Check sheet for the modelled part. Datum: model origin and axes. Units: mm. Coordinates: 2 decimals unless noted, no trailing zeros. Order: outer loops, then holes, each group sorted by start corner. A loop starts at its lowest first (then second) coordinate and runs counter-clockwise, first axis right, second up.
1. Cross-section at B-B (z = -17.75). Enter the section's corners in (x, y), then the cut area to 3 significant figures.
2. Cross-section at C-C (y = 0.75). Enter the section's corners in (x, z).
3. Gauge pin test, flat ends, axial feed: pin 1 Ø2 at (x, z) = (-12, 3.5) entering from -Y; pin 2 Ø1.2 at (x, y) = (1, 0.5) entering from +Z; pin 3 Ø2 at (y, z) = (3.5, -12) entering from +X; pin 4 Ø1.6 at (x, y) = (1, 1) entering from -Z. Record the tip position at first contact, or that the pin passes through.
4. Thickness scan on line 1 (Z direction, x = -33.5, y = 1.1); line 2 (X direction, y = 1, z = 0); line 3 (Z direction, x = -57.25, y = 2.9). Record the ranges inside material, lowest first.
5. Cross-section at D-D (x = -33.5). Enter the section's corners in (y, z).
6. Cross-section at A-A (x = -63.75). Enter the section's corners in (y, z).
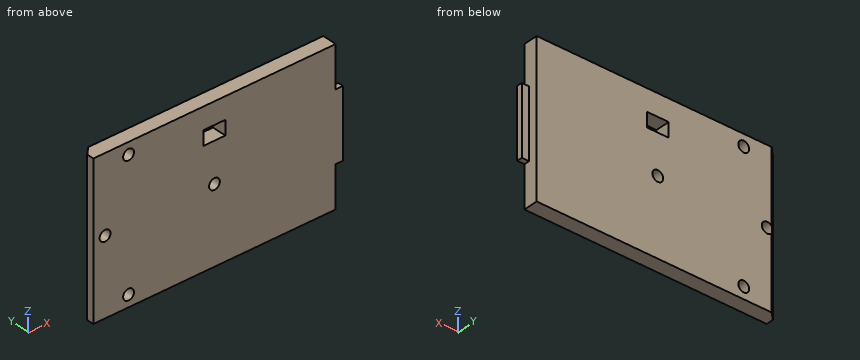
Autodesk Inventor part; units mm, degrees
ref_plane "YZ Plane" through (0, 0, 0) normal (1, 0, 0) x (0, 1, 0)
ref_plane "XZ Plane" through (0, 0, 0) normal (0, 1, 0) x (-1, 0, 0)
ref_plane "XY Plane" through (0, 0, 0) normal (0, 0, 1) x (1, 0, 0)
sketch "Sketch1" plane through (0, 0, 0) normal (0, 1, 0) x (-1, 0, 0)
  arc A0 (67, -23) -> (69, -21) centre (67, -21) ccw
  line L0 (69, -21) -> (69, 21)
  arc A1 (69, 21) -> (67, 23) centre (67, 21) ccw
  line L1 (67, 23) -> (0, 23)
  arc A2 (0, 23) -> (-2, 21) centre (0, 21) ccw
  line L2 (-2, 21) -> (-2, -21)
  arc A3 (-2, -21) -> (0, -23) centre (0, -21) ccw
  line L3 (0, -23) -> (67, -23)
  line L4 (67, -21) -> (0, -21)
  line L5 (0, -21) -> (0, 21)
  line L6 (0, 21) -> (67, 21)
  line L7 (67, 21) -> (67, -21)
  line L8 (67, 21) -> (60.5, 21)
  line L9 (60.5, 21) -> (60.5, 14.5)
  line L10 (60.5, 14.5) -> (67, 14.5)
  line L11 (67, 14.5) -> (67, 21)
  line L12 (67, -21) -> (67, 21)
  line L13 (67, -21) -> (60.5, -21)
  line L14 (60.5, -21) -> (60.5, -14.5)
  line L15 (60.5, -14.5) -> (67, -14.5)
  line L16 (67, -14.5) -> (67, -21)
  line L17 (67, -21) -> (60.5, -14.5)
  line L18 (67, 21) -> (69, 21)
  line L19 (67, 21) -> (60.5, 14.5)
  line L20 (0, 16.25) -> (-2, 16.25)
  circle A4 centre (64.5, -18.5) radius 1
  circle A5 centre (64.5, 18.5) radius 1
  line L21 (60.5, -21) -> (0, -21)
  line L22 (0, -21) -> (0, 21)
  line L23 (0, 21) -> (60.5, 21)
  line L24 (60.5, 21) -> (60.5, 14.5)
  line L25 (60.5, 14.5) -> (67, 14.5)
  line L26 (67, 14.5) -> (67, -14.5)
  line L27 (67, -14.5) -> (60.5, -14.5)
  line L28 (60.5, -14.5) -> (60.5, -21)
  arc A6 (67, -23) -> (69, -21) centre (67, -21) ccw
  line L29 (69, -21) -> (69, 21)
  arc A7 (69, 21) -> (67, 23) centre (67, 21) ccw
  line L30 (67, 23) -> (0, 23)
  arc A8 (0, 23) -> (-2, 21) centre (0, 21) ccw
  line L31 (-2, 21) -> (-2, -21)
  arc A9 (-2, -21) -> (0, -23) centre (0, -21) ccw
  line L32 (0, -23) -> (67, -23)
  line L33 (-2, -10) -> (0, -10)
  line L34 (0, -10) -> (0, 10)
  line L35 (0, 10) -> (-2, 10)
  line L36 (-2, 10) -> (-2, -10)
  line L37 (0, -21) -> (4.5, -21)
  line L38 (67, 21) -> (0, 21)
  line L39 (0, 21) -> (0, -21)
  line L40 (0, -21) -> (67, -21)
  line L41 (67, -21) -> (67, 21)
  line L42 (0, 16.25) -> (-2, 16.25)
  line L43 (67, -21) -> (60.5, -21)
  line L44 (0, -21) -> (0, 21)
  line L45 (0, 21) -> (54, 21)
  line L46 (67, 21) -> (67, 3.25)
  arc A10 (67, -23) -> (69, -21) centre (67, -21) ccw
  line L47 (69, -21) -> (69, 21)
  arc A11 (69, 21) -> (67, 23) centre (67, 21) ccw
  line L48 (67, 23) -> (0, 23)
  arc A12 (0, 23) -> (-2, 21) centre (0, 21) ccw
  line L49 (-2, 21) -> (-2, -21)
  arc A13 (-2, -21) -> (0, -23) centre (0, -21) ccw
  line L50 (0, -23) -> (67, -23)
  line L51 (-2, -10) -> (0, -10)
  line L52 (0, -10) -> (0, 10)
  line L53 (0, 10) -> (-2, 10)
  line L54 (-2, 10) -> (-2, -10)
  line L55 (0, -21) -> (4.5, -21)
  line L56 (67, 21) -> (0, 21)
  line L57 (0, 21) -> (0, -21)
  line L58 (0, -21) -> (67, -21)
  line L59 (67, -21) -> (67, 21)
  line L60 (60.5, -21) -> (60.5, -14.5)
  line L61 (60.5, -14.5) -> (54, -14.5)
  line L62 (54, -14.5) -> (54, -21)
  line L63 (54, -21) -> (0, -21)
  line L64 (54, 21) -> (54, 14.5)
  line L65 (54, 14.5) -> (60.5, 14.5)
  line L66 (60.5, 14.5) -> (60.5, 21)
  line L67 (60.5, 21) -> (67, 21)
  line L68 (67, 3.25) -> (60.5, 3.25)
  line L69 (60.5, 3.25) -> (60.5, -3.25)
  line L70 (60.5, -3.25) -> (67, -3.25)
  line L71 (67, -3.25) -> (67, -21)
  line L72 (67, -3.25) -> (60.5, 3.25)
  line L73 (54, -14.5) -> (60.5, -21)
  line L74 (54, 14.5) -> (60.5, 21)
  point P0 (0, 0)
  point P1 (0, 0)
  point P2 (0, 0)
  point P3 (0, 0)
  point P4 (63.75, 0)
  point P5 (57.25, -17.75)
  point P6 (57.25, 17.75)
  dimension "d0" = 6.5
  dimension "d1" = 6.5
  dimension "d2" = 6.5
  dimension "d3" = 6.5
  dimension "d4" = 10
  dimension "d5" = 10
  dimension "d25" = 10
  dimension "d26" = 10
extrude "Extrusion1" add sketch "Sketch1" along normal blind 2 contours L19 A5 L9 L6 | L7 L10 L19 A5 | L2 L35 L5 L33 | L74 L64 L6 | L9 L65 L74 | L7 L68 L69 L70 L15 L61 L62 L4 L5 L6 L64 L65 L10 | A5 L19 | L19 A5 | L7 L72 L68 | L70 L69 L72 | L7 L17 A4 L15 | L62 L73 L4 | L4 L14 L17 A4 | L14 L73 L61 | A4 L17 | L17 A4
sketch "Sketch2" plane through (0, 2, 0) normal (0, 1, 0) x (1, 0, 0)
  line L0 (0, -10) -> (2, -10)
  line L1 (2, -10) -> (2, 10)
  line L2 (2, 10) -> (0, 10)
  line L3 (0, 10) -> (0, 21)
  line L4 (0, 21) -> (-67, 21)
  line L5 (-67, 21) -> (-67, -21)
  line L6 (-67, -21) -> (0, -21)
  line L7 (0, -21) -> (0, -10)
  line L8 (-67, -21) -> (0, -21)
  line L9 (0, -21) -> (0, 21)
  line L10 (0, 21) -> (-67, 21)
  line L11 (-67, 21) -> (-67, -21)
  point P0 (0, 0)
extrude "Extrusion2" add sketch "Sketch2" along normal blind 2 contours L7 L6 L5 L4 L3 L9
sketch "Sketch3" plane through (-67, 0, 21) normal (0, 0, 1) x (1, 0, 0)
  point P0 (67, 0)
sketch "Sketch4" plane through (0, 4, 0) normal (0, 1, 0) x (1, 0, 0)
  line L0 (0, 21) -> (-67, 21)
  line L1 (-67, 21) -> (-67, -21)
  line L2 (-67, -21) -> (0, -21)
  line L3 (0, -21) -> (0, 21)
  line L4 (0, 10) -> (0, 21)
  line L5 (0, 21) -> (-67, -21)
  point P0 (0, 0)
  point P1 (-33.5, 0)
  point P2 (-57.25, 17.75)
  point P3 (-63.75, 0)
  point P4 (-57.25, -17.75)
  point P5 (-57.25, 17.75)
  point P6 (-63.75, 0)
  point P7 (-57.25, -17.75)
hole "Hole1" at (-33.5, 4, 0) at (-57.25, 4, -17.75) at (-57.25, 4, 17.75) at (-63.75, 4, 0) direction (0, -1, 0) diameter 3 depth 8 tip angle 118
sketch "Sketch5" plane through (2, 0, 10) normal (1, 0, 0) x (0, 0, -1)
  line L0 (0, 0) -> (20, 0)
  line L1 (20, 0) -> (20, 2)
  line L2 (0, 2) -> (20, 2)
  line L3 (0, 0) -> (0, 2)
  line L4 (20, 2) -> (20, 0)
  line L5 (20, 0) -> (0, 0)
  line L6 (0, 0) -> (0, 2)
  line L7 (0, 2) -> (20, 2)
  line L8 (0, 0) -> (20, 0)
  line L9 (0.5, 0) -> (19.5, 0)
  line L10 (19.5, 0) -> (19.5, 1.5)
  line L11 (19.5, 1.5) -> (0.5, 1.5)
  line L12 (0.5, 1.5) -> (0.5, 0)
  point P0 (10, 0)
  dimension "d20" = 0.5
  dimension "d21" = 0.5
  dimension "d22" = 0.5
extrude "Extrusion4" cut sketch "Sketch5" against normal up to surface (2 mm away) contours L3 L2 L1 L0 L10 L11 L12
sketch "Sketch6" plane through (0, 0, 0) normal (0, -1, 0) x (1, 0, 0)
  line L0 (-30.5, 15) -> (-36.5, 15)
  line L1 (-36.5, 15) -> (-36.5, 11)
  line L2 (-36.5, 11) -> (-30.5, 11)
  line L3 (-30.5, 11) -> (-30.5, 15)
  circle A0 centre (-63.75, 0) radius 1.5
  circle A1 centre (-57.25, -17.75) radius 1.5
  circle A2 centre (-33.5, 0) radius 1.5
  circle A3 centre (-57.25, 17.75) radius 1.5
  line L4 (2, 9.5) -> (0, 9.5)
  line L5 (0, 21) -> (0, 9.5)
  line L6 (-67, 21) -> (0, 21)
  line L7 (-67, -21) -> (-67, 21)
  line L8 (0, -21) -> (-67, -21)
  line L9 (0, -21) -> (0, -9.5)
  line L10 (0, -9.5) -> (2, -9.5)
  line L11 (2, 9.5) -> (2, -9.5)
  line L12 (-33.5, 21) -> (-33.5, 15)
  point P0 (0, 0)
  dimension "d27" = 4
  dimension "d28" = 6
  dimension "d29" = 6
extrude "Extrusion5" cut sketch "Sketch6" against normal through all contours L3 L2 L1 L0
chamfer "Chamfer1" distance 2 angle 45 1 edges at (-67, 4, 0)
properties part number "ttgorear"
Data:
1. outline: (-67, 0) - (-58.75, 0) - (-58.75, 4) - (-65, 4) - (-67, 2) - close; (-55.75, 0) - (0, 0) - (0, 4) - (-55.75, 4) - close
1. area: 254 mm2
2. outline: (-67, -21) - (0, -21) - (0, -9.5) - (2, -9.5) - (2, 9.5) - (0, 9.5) - (0, 21) - (-67, 21) - close; hole circle Ø3 at (-63.75, 0); hole circle Ø3 at (-57.25, -17.75); hole circle Ø3 at (-57.25, 17.75); hole (-36.5, 11) - (-30.5, 11) - (-30.5, 15) - (-36.5, 15) - close; hole circle Ø3 at (-33.5, 0)
3. pin 1: stops at y = 0
3. pin 2: stops at z = 9.5
3. pin 3: stops at x = 0
3. pin 4: stops at z = -9.5
4. line 1: z = -21 to -1.5, 1.5 to 11, 15 to 21
4. line 2: x = -67 to -65.25, -62.25 to -35, -32 to 2
4. line 3: z = -21 to -19.25, -16.25 to 16.25, 19.25 to 21
5. outline: (0, -21) - (4, -21) - (4, -1.5) - (0, -1.5) - close; (0, 1.5) - (4, 1.5) - (4, 11) - (0, 11) - close; (0, 15) - (4, 15) - (4, 21) - (0, 21) - close
6. outline: (0, -21) - (4, -21) - (4, -1.5) - (0, -1.5) - close; (0, 1.5) - (4, 1.5) - (4, 21) - (0, 21) - close
